Geometry: see drawing. Coordinates: mm, zero at the bounding-box minimum. Coordinates: 2 decimals unless noted, no trailing zeros. Order: outer loops, then holes, each group sorted by start corner. A loop starts at its lowest first (then second) coordinate and runs counter-clockwise, first axis right, second up.
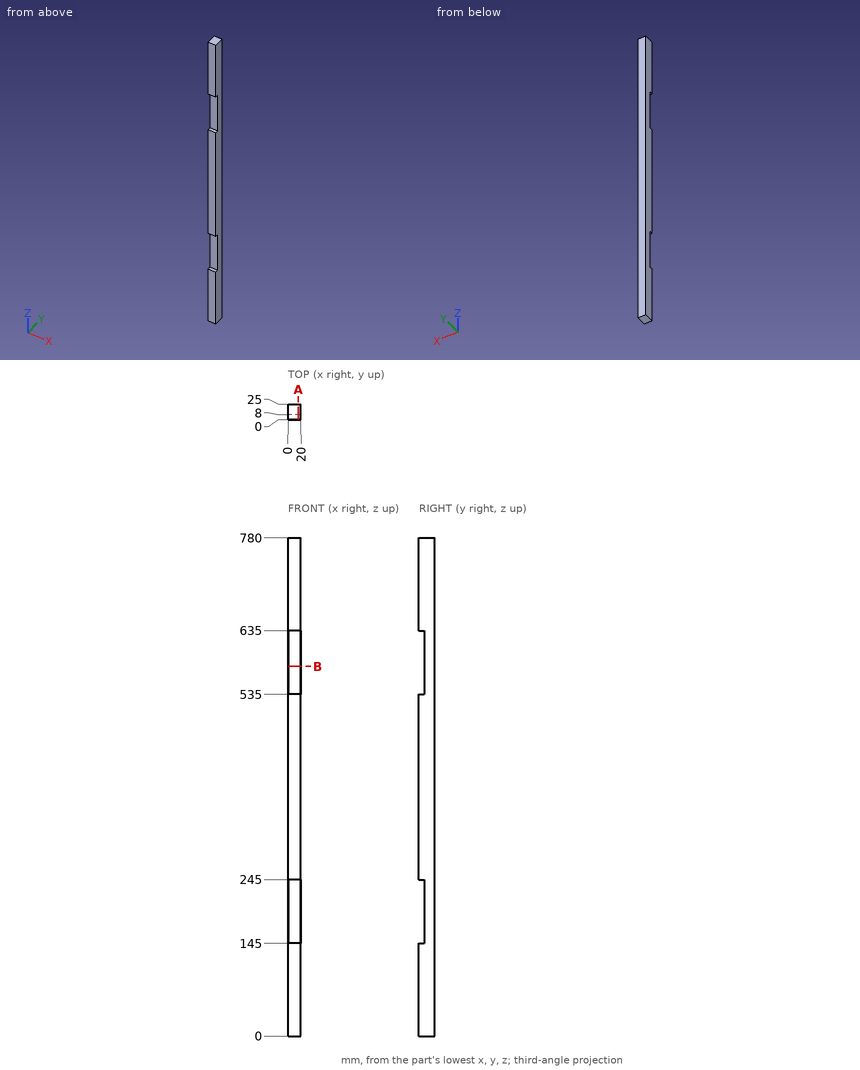
Item 1: Pin query (flat end, axial travel): pin 1 Ø1.5 at (x, z) = (5, 238.5) entering from -Y. Return the tip coordinate at first contact, or that it passes through.
Response values:
pin 1: stops at y = 8
Item 2: Cut plane A-A on x = 16. Return loops of the section in (y, z), then the cut area to 3 significant figures.
Response values:
outline: (0, 0) - (25, 0) - (25, 780) - (0, 780) - (0, 635) - (8, 635) - (8, 535) - (0, 535) - (0, 245) - (8, 245) - (8, 145) - (0, 145) - close
area: 17,900 mm2
Item 3: Cut plane B-B on z = 579. Return loops of the section in (x, y), then the cut area to 3 significant figures.
Response values:
outline: (0, 8) - (20, 8) - (20, 25) - (0, 25) - close
area: 340 mm2
Item 4: Ray query, probe 1 along Z at (x, y) = (16.25, 5.75); probe 2 along Y at (x, z) = (14.25, 604). Return the intervals inside material, ascending.
Response values:
probe 1: z = 0 to 145, 245 to 535, 635 to 780
probe 2: y = 8 to 25
